Design review of the part built by this model. Coordinates are the model's own, in mm. A direction names the side the tool comes from. Coordinates: 2 decimals unless noted, no trailing zeros. Write each loop counter-clockwise with the first axis right and the second up, starting at its lowest first coordinate (ties: lowest second). Pieces come first, ordered by that corner, then holes.
Q1. For probe 1 along Y at (x, z) = (-19, 8); probe 2 along Z at (x, y) = (-26, -12); probe 3 along X at (y, z) = (-4, 32), list the stretches that pass through material, from the lowest coordinate up.
Q2. Take a section at A-A (y = 4.5). Give the boundary of the cut face in (x, z), and give its area (3 significant figures).
Q3. Take a section at B-B (z = 7). Give the boundary of the cut face in (x, y), and give its area (3 significant figures).
Q4. Mouldability with a two-part tool opening along Y and no side actions: class faces 1 (the flat face through (-5, 24.702, 6)), 2 (the cylindrical face through (55.885, 5.503, 18.783)), 3 (the flat face through (-13, 0, 12.7)) as pulls with the +Y half, pulls with the -Y half, needs draft (parallel to the pull), parting line crosses it, or undercut.
Q5. Take a section at D-D (y = -9). Give the boundary of the cut face in (x, z).
Q6. Take a section at C-C (x = 0.5). Give the boundary of the cut face in (y, z).
Q7. Insertion check: pin 1 (17.5 mm diameter, centred on x = -1, z = 17.5, fed in from -Y); pin 2 (17.5 mm diameter, centred on x = 3.5, z = 17.5, fed in from +Y); pin 3 (12 mm diameter, centred on y = -8, z = 26.5, fed in from -X); pin 4 (6 mm diameter, centred on x = 45, y = -12, fed in from +Z). Each pin has a flat end and moves straight along its axis. Give the tip position at first contact, or say it passes through.
Q8. Machinability: for faces 4 (the flat face through (5, 6.35, 17)), 5 (the flat face through (-6, -24.702, 6)), 6 (the flat face through (5, -6.35, 17)), 7 (the flat face through (44, -18, 38.1)), which of the approach directions +Z, -Z, +X, -X, +Y, -Y give a long, thin tool a straight path to every point of the face, cutting with its end or side? Answer none if there is none.
```python
from build123d import *

# Parameters (mm, degrees)
F0_R     = 18.321779
F1_DEPTH = 38.1
F2_DEPTH = 12.7
F4_DEPTH = 6.35


with BuildPart() as f1:
    # F0 (on Top) → F1 (new body)
    with BuildSketch(Plane.XY):
        with BuildLine():
            ThreePointArc((65.62934, 0), (53.067244, 22.936208), (26.97591, 24.702042))
            ThreePointArc((26.97591, 24.702042), (11.189707, 0), (26.97591, -24.702042))
            ThreePointArc((26.97591, -24.702042), (53.067244, -22.936208), (65.62934, 0))
        make_face()
        with Locations((38.409524, 0)):
            Circle(F0_R, mode=Mode.SUBTRACT)
    extrude(amount=F1_DEPTH)

    # F0 (on Top) → F2 (join)
    with BuildSketch(Plane.XY):
        with BuildLine():
            ThreePointArc((26.97591, -24.702042), (11.189707, 0), (26.97591, 24.702042))
            Line((26.97591, 24.702042), (-38.409524, 24.702042))
            Line((-38.409524, 24.702042), (-38.409524, -24.702042))
            Line((-38.409524, -24.702042), (26.97591, -24.702042))
        make_face()
    extrude(amount=F2_DEPTH)

    # F3 (on Front) → F4 (join, symmetric)
    with BuildSketch(Plane.XZ):
        Polygon((14.299882, 9.182032), (14.299882, 30.255545), (-17.310385, 9.182032), align=None)
    extrude(amount=F4_DEPTH, both=True)


solid = f1.part
```
Response:
1. probe 1: y = -24.7 to 24.7
1. probe 2: z = 0 to 12.7
1. probe 3: x = 11.49 to 20.53, 56.29 to 65.33
2. outline: (-38.41, 0) - (20.65, 0) - (20.65, 38.1) - (11.56, 38.1) - (11.56, 28.43) - (-12.03, 12.7) - (-38.41, 12.7) - close; (56.17, 0) - (65.25, 0) - (65.25, 38.1) - (56.17, 38.1) - close
2. area: 1,510 mm2
3. outline: (-38.41, -24.7) - (26.98, -24.7) arc R27.22 ccw (long way) to (26.98, 24.7) - (-38.41, 24.7) - close; hole circle Ø36.64 at (38.41, 0)
3. area: 3,940 mm2
4. face 1: pulls with the +Y half
4. face 2: undercut
4. face 3: needs draft
5. outline: (-38.41, 0) - (22.45, 0) - (22.45, 38.1) - (12.72, 38.1) - (12.72, 12.7) - (-38.41, 12.7) - close; (54.37, 0) - (64.1, 0) - (64.1, 38.1) - (54.37, 38.1) - close
6. outline: (-24.7, 0) - (24.7, 0) - (24.7, 12.7) - (6.35, 12.7) - (6.35, 21.06) - (-6.35, 21.06) - (-6.35, 12.7) - (-24.7, 12.7) - close
7. pin 1: stops at y = -24.7
7. pin 2: stops at y = 24.7
7. pin 3: stops at x = 0.01
7. pin 4: passes through
8. face 4: +Z, -X, +Y
8. face 5: +Z, -Z, -X, -Y
8. face 6: +Z, -X, -Y
8. face 7: +Z, +X, -X, +Y, -Y
